Input: part model. Units: mm. Frame: model coordinates. A direction names the side the tool comes from. Round coordinates to 2 decimals unless told otherwise and drop trailing zeros. Loops run counter-clockwise (first coordinate to the right, second up) from the corner with the lowest first, then second, coordinate; pieces in that order, holes last. Notation, with made-up numbers: M 83,52.5 L 109,52.5 A24 cw 109,88.5 Z; hole C -36.5,52.5 d9. An arc over 180 degrees is marked long. Put each result on its own line as item: value. Start each with the question number.
1) Section D-D on x = -25. Output: boundary loops of the cut face in (y, z), plus the area to 3 significant figures.
2) Pin query (flat end, axial travel): pin 1 (4 mm diameter, centred on x = 11.5, z = -41, fed in from +Y); pin 2 (0.8 mm diameter, centred on y = 6.5, z = 17.5, fed in from +X); pin 3 (2 mm diameter, centred on x = -25, z = -36, fed in from -Y); pin 4 (1.2 mm diameter, centred on x = -0.5, y = 6, fed in from -Z). Return the tip coordinate at first contact, or that it passes through.
3) Line query: probe 1 along X at (y, z) = (1.45, -36); probe 2 along X at (y, z) = (11, -5); probe 3 along Z at (x, y) = (23.5, 2.5). Output: solid intervals per line, ascending.
4) Section C-C on z = -4.5. Output: boundary loops of the cut face in (x, y), plus the area to 3 significant figures.
5) Section B-B on x = -5.5. Output: boundary loops of the cut face in (y, z).
6) Reachability of faces 1 (the face through (0.4, 5, -17.4)), 2 (the face through (38, 2, -4)), 3 (the face through (22.5, 3, -5)) from +Z, -Z, +X, -X, +Y, -Y: full face, straight path, thin tool, end or side. Return the list, or none.
7) Section A-A on z = 41. Output: boundary loops of the cut face in (x, y), plus the area to 3 significant figures.
8) Draft query along Z for faces 4 (the face through (33.794, 1.521, -53.973)), 5 (the face through (0, 7.5, -28)), 6 (the face through (-1, 0, -28)). Return one class per face: +Z half, -Z half, draft (parallel to the pull), parting line (faces both ways), or undercut.
from build123d import *

# Parameters (mm, degrees)
SKETCH1_W                  = 60
SKETCH1_H                  = 102
BOSS_EXTRUDE1_DEPTH        = 3
M3_CLEARANCE_HOLE1_D       = 3.4
SKETCH5_R                  = 35
BOSS_EXTRUDE2_DEPTH        = 10
SKETCH6_R                  = 27
CUT_EXTRUDE1_DEPTH         = 8
SKETCH8_W                  = 5
SKETCH8_H                  = 5.5
BOSS_EXTRUDE3_DEPTH        = 2.5
SKETCH9_W                  = 5
SKETCH9_H                  = 5
BOSS_EXTRUDE4_DEPTH        = 2.5
SKETCH10_W                 = 45
SKETCH10_H                 = 24
CUT_EXTRUDE2_DEPTH         = 63.369864518
SKETCH12_W                 = 60
SKETCH12_H                 = 2
CUT_EXTRUDE3_DEPTH         = 63.657800791
SKETCH13_W                 = 60
SKETCH13_H                 = 3
CUT_EXTRUDE4_DEPTH         = 63.657800791
SKETCH14_W                 = 60
SKETCH14_H                 = 3
BOSS_EXTRUDE5_DEPTH        = 9
SKETCH16_W                 = 106
SKETCH16_H                 = 3
BOSS_EXTRUDE6_DEPTH        = 8
SKETCH17_W                 = 106
SKETCH17_H                 = 3
BOSS_EXTRUDE7_DEPTH        = 8
CUT_EXTRUDE5_DEPTH         = 15
CUT_EXTRUDE6_DEPTH         = 71.057119553
M3X0_5_TAPPED_HOLE1_REACH  = 102.233
M3X0_5_TAPPED_HOLE1_BORE_R = 1.25
M3X0_5_TAPPED_HOLE2_REACH  = 102.233
M3X0_5_TAPPED_HOLE2_BORE_R = 1.25
M3X0_5_TAPPED_HOLE3_REACH  = 98.284
M3X0_5_TAPPED_HOLE3_BORE_R = 1.25
SKETCH28_W                 = 76
SKETCH28_H                 = 1.5
CUT_EXTRUDE7_DEPTH         = 71.057119567


with BuildPart() as part:
    # Sketch1 → Boss-Extrude1 (new body)
    with BuildSketch(Plane(origin=(0, 0, 0), x_dir=(1, 0, 0), z_dir=(0, 1, 0))):
        Rectangle(SKETCH1_W, SKETCH1_H)
    extrude(amount=BOSS_EXTRUDE1_DEPTH)

    # M3 Clearance Hole1 (through all)
    with Locations(Plane(origin=(-25, 3, -36), x_dir=(0, 0, 1), z_dir=(0, 1, 0))):
        with Locations((0, 0), (0, 50), (77, 0), (77, 50)):
            Hole(M3_CLEARANCE_HOLE1_D / 2)

    # Sketch5 → Boss-Extrude2 (add)
    with BuildSketch(Plane(origin=(0, 3, 0), x_dir=(1, 0, 0), z_dir=(0, 1, 0))):
        with Locations(Location((0, 5, 0), (0, 0, 148.997280866))):
            Circle(SKETCH5_R)
    extrude(amount=BOSS_EXTRUDE2_DEPTH)

    # Sketch6 → Cut-Extrude1 (cut)
    with BuildSketch(Plane(origin=(0, 13, 0), x_dir=(1, 0, 0), z_dir=(0, 1, 0))):
        with Locations(Location((0, 5, 0), (0, 0, 270))):
            Circle(SKETCH6_R)
    extrude(amount=-CUT_EXTRUDE1_DEPTH, mode=Mode.SUBTRACT)

    # Sketch8 → Boss-Extrude3 (add)
    with BuildSketch(Plane(origin=(0, 5, 0), x_dir=(1, 0, 0), z_dir=(0, 1, 0))):
        with Locations((0, 27.5)):
            Rectangle(SKETCH8_W, SKETCH8_H)
    extrude(amount=BOSS_EXTRUDE3_DEPTH)

    # Sketch9 → Boss-Extrude4 (add)
    with BuildSketch(Plane(origin=(0, 5, 0), x_dir=(1, 0, 0), z_dir=(0, 1, 0))):
        with Locations((0, -17)):
            Rectangle(SKETCH9_W, SKETCH9_H)
    extrude(amount=BOSS_EXTRUDE4_DEPTH)

    # Sketch10 → Cut-Extrude2 (cut, through all)
    with BuildSketch(Plane(origin=(0, 5, 0), x_dir=(1, 0, 0), z_dir=(0, 1, 0))):
        with Locations((0, 5)):
            Rectangle(SKETCH10_W, SKETCH10_H)
    extrude(amount=-CUT_EXTRUDE2_DEPTH, mode=Mode.SUBTRACT)

    # Sketch12 → Cut-Extrude3 (cut, through all)
    with BuildSketch(Plane(origin=(0, 3, 0), x_dir=(1, 0, 0), z_dir=(0, 1, 0))):
        with Locations((0, 50)):
            Rectangle(SKETCH12_W, SKETCH12_H)
    extrude(amount=-CUT_EXTRUDE3_DEPTH, mode=Mode.SUBTRACT)

    # Sketch13 → Cut-Extrude4 (cut, through all)
    with BuildSketch(Plane(origin=(0, 3, 0), x_dir=(1, 0, 0), z_dir=(0, 1, 0))):
        with Locations((0, -49.5)):
            Rectangle(SKETCH13_W, SKETCH13_H)
    extrude(amount=-CUT_EXTRUDE4_DEPTH, mode=Mode.SUBTRACT)

    # Sketch14 → Boss-Extrude5 (add)
    with BuildSketch(Plane(origin=(0, 0, -49), x_dir=(-1, 0, 0), z_dir=(0, 0, -1))):
        with Locations((0, 1.5)):
            Rectangle(SKETCH14_W, SKETCH14_H)
    extrude(amount=BOSS_EXTRUDE5_DEPTH)

    # Sketch16 → Boss-Extrude6 (add)
    with BuildSketch(Plane.ZY.offset(30)):
        with Locations((-5, 1.5)):
            Rectangle(SKETCH16_W, SKETCH16_H)
    extrude(amount=BOSS_EXTRUDE6_DEPTH)

    # Sketch17 → Boss-Extrude7 (add)
    with BuildSketch(Plane(origin=(30, 0, 0), x_dir=(0, 0, -1), z_dir=(1, 0, 0))):
        with Locations((5, 1.5)):
            Rectangle(SKETCH17_W, SKETCH17_H)
    extrude(amount=BOSS_EXTRUDE7_DEPTH)

    # Sketch18 → Cut-Extrude5 (cut)
    with BuildSketch(Plane(origin=(0, 3, 0), x_dir=(1, 0, 0), z_dir=(0, 1, 0))):
        with BuildLine():
            Line((38, 46), (38, 58))
            Line((38, 58), (26, 58))
            ThreePointArc((26, 58), (33.884200012, 53.884200012), (38, 46))
        make_face()
    extrude(amount=-CUT_EXTRUDE5_DEPTH, mode=Mode.SUBTRACT)

    # Sketch19 → Cut-Extrude6 (cut, through all)
    with BuildSketch(Plane(origin=(0, 3, 0), x_dir=(1, 0, 0), z_dir=(0, 1, 0))):
        with BuildLine():
            Line((38, -36), (38, -48))
            Line((38, -48), (26, -48))
            ThreePointArc((26, -48), (33.934883201, -43.934883201), (38, -36))
        make_face()
    extrude(amount=-CUT_EXTRUDE6_DEPTH, mode=Mode.SUBTRACT)

    # M3x0.5 Tapped Hole1 bore (on position points) → M3x0.5 Tapped Hole1 (cut, up to next)
    with BuildSketch(Plane(origin=(-14.832396974, 9, -36.701734968), x_dir=(-0.905763856237, 0, 0.423782770691), z_dir=(-0.423782770691, 0, -0.905763856237)), mode=Mode.PRIVATE) as m3x0_5_tapped_hole1_sk1:
        Circle(M3X0_5_TAPPED_HOLE1_BORE_R)
    m3x0_5_tapped_hole1_tool1 = extrude(m3x0_5_tapped_hole1_sk1.sketch, amount=-M3X0_5_TAPPED_HOLE1_REACH, mode=Mode.PRIVATE) & part.part
    add(m3x0_5_tapped_hole1_tool1.solids().sort_by_distance((-14.832397, 9, -36.701735))[0], mode=Mode.SUBTRACT)

    # M3x0.5 Tapped Hole2 bore (on position points) → M3x0.5 Tapped Hole2 (cut, up to next)
    with BuildSketch(Plane(origin=(14.832396974, 9, -36.701734968), x_dir=(-0.905763856237, 0, -0.423782770691), z_dir=(0.423782770691, 0, -0.905763856237)), mode=Mode.PRIVATE) as m3x0_5_tapped_hole2_sk1:
        Circle(M3X0_5_TAPPED_HOLE2_BORE_R)
    m3x0_5_tapped_hole2_tool1 = extrude(m3x0_5_tapped_hole2_sk1.sketch, amount=-M3X0_5_TAPPED_HOLE2_REACH, mode=Mode.PRIVATE) & part.part
    add(m3x0_5_tapped_hole2_tool1.solids().sort_by_distance((14.832397, 9, -36.701735))[0], mode=Mode.SUBTRACT)

    # M3x0.5 Tapped Hole3 bore (on position points) → M3x0.5 Tapped Hole3 (cut, up to next)
    with BuildSketch(Plane(origin=(0.02, 9, 29.999994286), x_dir=(0.999999836735, 0, -0.000571428571), z_dir=(0.000571428571, 0, 0.999999836735)), mode=Mode.PRIVATE) as m3x0_5_tapped_hole3_sk1:
        Circle(M3X0_5_TAPPED_HOLE3_BORE_R)
    m3x0_5_tapped_hole3_tool1 = extrude(m3x0_5_tapped_hole3_sk1.sketch, amount=-M3X0_5_TAPPED_HOLE3_REACH, mode=Mode.PRIVATE) & part.part
    add(m3x0_5_tapped_hole3_tool1.solids().sort_by_distance((0.02, 9, 29.999994))[0], mode=Mode.SUBTRACT)

    # Sketch28 → Cut-Extrude7 (cut, through all)
    with BuildSketch(Plane(origin=(0, 3, 0), x_dir=(1, 0, 0), z_dir=(0, 1, 0))):
        with Locations((0, -47.25)):
            Rectangle(SKETCH28_W, SKETCH28_H)
    extrude(amount=-CUT_EXTRUDE7_DEPTH, mode=Mode.SUBTRACT)


solid = part.part
Geometry results:
1. outline: M 0,-58 L 3,-58 L 3,-37.7 L 0,-37.7 Z; M 0,-34.3 L 3,-34.3 L 3,-29.49 L 13,-29.49 L 13,-15.2 L 5,-15.2 L 5,5.2 L 13,5.2 L 13,19.49 L 3,19.49 L 3,39.3 L 0,39.3 Z; M 0,42.7 L 3,42.7 L 3,46.5 L 0,46.5 Z
1. area: 620 mm²
2. pin 1: stops at y = 3
2. pin 2: stops at x = 27.14
2. pin 3: passes through
2. pin 4: stops at z = -40
3. probe 1: x = -38 to -26.7, -23.3 to 23.3, 26.7 to 38
3. probe 2: x = -35 to -27, 27 to 35
3. probe 3: z = -58 to -36.8, -35.2 to 40.2, 41.8 to 46.5
4. outline: M -38,0 L -22.5,0 L -22.5,5 L -27,5 L -27,13 L -35,13 L -35,3 L -38,3 Z; M 22.5,0 L 38,0 L 38,3 L 35,3 L 35,13 L 27,13 L 27,5 L 22.5,5 Z
4. area: 271 mm²
5. outline: M 0,-58 L 3,-58 L 3,-39.57 L 13,-39.57 L 13,-31.43 L 5,-31.43 L 5,-17 L 0,-17 Z; M 0,7 L 5,7 L 5,21.43 L 13,21.43 L 13,29.57 L 3,29.57 L 3,46.5 L 0,46.5 Z
6. face 1: +Y
6. face 2: +Z, -Z, +X, +Y, -Y
6. face 3: +Y, -Y
7. outline: M -38,0 L -26.7,0 L -26.7,3 L -38,3 Z; M -23.3,0 L 23.3,0 L 23.3,3 L -23.3,3 Z; M 26.7,0 L 36.2,0 L 36.2,3 L 26.7,3 Z
7. area: 202 mm²
8. face 4: -Z half
8. face 5: undercut
8. face 6: draft
